Could you check a few things on this model? Use its own coordinates, in mm. Face numbers are marked on the shaded views. Round coordinates to 2 decimals unless told otherwise and drop trailing zeros. Write each loop counter-clockwise with the first axis right and the second up, starting at its lowest first coordinate (ties: lowest second). Pieces come first, ordered by that corner, then holes. Notation, with made-up numbers: M 30.25,-22 L 80.25,-22 A19 ccw 80.25,2 Z; hole C -11,-19 d3. An arc over 180 degrees is marked long. One line per question, with ' | ' between items. Start each with the question number.
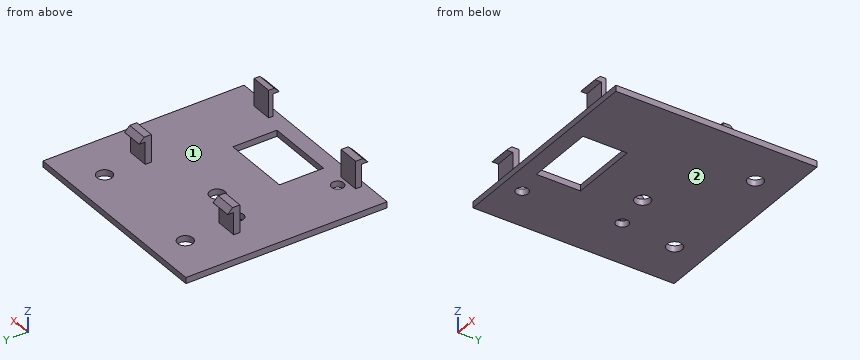
```python
from build123d import *

# Parameters (mm, degrees)
SKETCH_W        = 69
SKETCH_H        = 66
SKETCH_R        = 2.5
SKETCH_R_2      = 2
SKETCH_W_2      = 22.5
SKETCH_H_2      = 14.5
PAD_DEPTH       = 2
SKETCH011_R     = 2.5
POCKET_DEPTH    = 2
SKETCH012_W     = 7
SKETCH012_H     = 2
SKETCH012_H_2   = 1.5
PAD001_DEPTH    = 9
SKETCH013_W     = 7
SKETCH013_H     = 1.7
PAD002_DEPTH    = 2
CHAMFER_SIZE    = 1.65
SKETCH014_W     = 7
SKETCH014_H     = 1.7
PAD003_DEPTH    = 2
CHAMFER001_SIZE = 1.65
SKETCH015_W     = 7
SKETCH015_H     = 1.7
PAD004_DEPTH    = 2
CHAMFER002_SIZE = 1.65
SKETCH016_W     = 7
SKETCH016_H     = 1.7
PAD005_DEPTH    = 2
CHAMFER003_SIZE = 1.65


with BuildPart() as part:
    # Sketch → Pad (new body)
    with BuildSketch(Plane.XY):
        Rectangle(SKETCH_W, SKETCH_H)
        with Locations((-19.5, 23)):
            Circle(SKETCH_R, mode=Mode.SUBTRACT)
        with Locations((19.5, 23)):
            Circle(SKETCH_R, mode=Mode.SUBTRACT)
        with Locations((-20.25, -26.5)):
            Circle(SKETCH_R_2, mode=Mode.SUBTRACT)
        with Locations((-17.85, 4.7)):
            Circle(SKETCH_R_2, mode=Mode.SUBTRACT)
        with Locations((0, -20.75)):
            Rectangle(SKETCH_W_2, SKETCH_H_2, mode=Mode.SUBTRACT)
    extrude(amount=PAD_DEPTH)

    # Sketch011 → Pocket (cut)
    with BuildSketch(Plane.XY.offset(2)):
        with Locations((-5.5, 3)):
            Circle(SKETCH011_R)
    extrude(amount=-POCKET_DEPTH, mode=Mode.SUBTRACT)

    # Sketch012 (on Face5 of Pocket) → Pad001 (join)
    with BuildSketch(Plane.XY.offset(2)):
        with Locations((-21, 9.5)):
            Rectangle(SKETCH012_W, SKETCH012_H)
        with Locations((21, -30.25)):
            Rectangle(SKETCH012_W, SKETCH012_H_2)
        with Locations((21, 10)):
            Rectangle(SKETCH012_W, SKETCH012_H)
        with Locations((-21, -30.5)):
            Rectangle(SKETCH012_W, SKETCH012_H)
    extrude(amount=PAD001_DEPTH)

    # Sketch013 (on Face22 of Pad001) → Pad002 (join)
    with BuildSketch(Plane.XZ.offset(31.5)):
        with Locations((-21, 10.15)):
            Rectangle(SKETCH013_W, SKETCH013_H)
    extrude(amount=PAD002_DEPTH)

    # Chamfer
    chamfer_edges = [part.edges().sort_by_distance(p)[0] for p in [
        (-21, -33.5, 11),
    ]]
    chamfer(chamfer_edges, length=CHAMFER_SIZE)

    # Sketch014 (on Face32 of Chamfer) → Pad003 (join)
    with BuildSketch(Plane.XZ.offset(31)):
        with Locations((21, 10.15)):
            Rectangle(SKETCH014_W, SKETCH014_H)
    extrude(amount=PAD003_DEPTH)

    # Chamfer001
    chamfer001_edges = [part.edges().sort_by_distance(p)[0] for p in [
        (21, -33, 11),
    ]]
    chamfer(chamfer001_edges, length=CHAMFER001_SIZE)

    # Sketch015 (on Face16 of Pad001) → Pad004 (join)
    with BuildSketch(Plane(origin=(0, 11, 0), x_dir=(-1, 0, 0), z_dir=(0, 1, 0))):
        with Locations((-21, 10.15)):
            Rectangle(SKETCH015_W, SKETCH015_H)
    extrude(amount=PAD004_DEPTH)

    # Chamfer002
    chamfer002_edges = [part.edges().sort_by_distance(p)[0] for p in [
        (21, 13, 11),
    ]]
    chamfer(chamfer002_edges, length=CHAMFER002_SIZE)

    # Sketch016 (on Face24 of Chamfer002) → Pad005 (join)
    with BuildSketch(Plane(origin=(0, 10.5, 0), x_dir=(-1, 0, 0), z_dir=(0, 1, 0))):
        with Locations((21, 10.15)):
            Rectangle(SKETCH016_W, SKETCH016_H)
    extrude(amount=PAD005_DEPTH)

    # Chamfer003
    chamfer003_edges = [part.edges().sort_by_distance(p)[0] for p in [
        (-21, 12.5, 11),
    ]]
    chamfer(chamfer003_edges, length=CHAMFER003_SIZE)


solid = part.part
```
1. Suppose I cut it at A-A (z = 3.75). Write out the boundary of the cut face in (x, y).
2. Suppose I cut it at C-C (y = -16.5). Write out the boundary of the cut face in (x, z).
3. If we mould it in two halves opening along Y, with no side actions, what happens to the marked faces 1 and 2? For each: released by +Y, released by -Y, zero draft, split by the parting line, or undercut.
4. Suppose I cut it at D-D (x = 19.5). Write out the boundary of the cut face in (y, z), and give its area (3 significant figures).
5. I'm going to push flat-ended pins straight in: P1, Ø3.5, axis at x = -19.5, z = 5.5, coming from the +Y side; P2, Ø3, axis at y = -32, z = 6, coming from the +X side; P3, Ø4, axis at x = 26.5, z = 2.5, coming from the -Y side. Where does each tip first touch, or does it pass through?
6. I need wall thicknesses on line 1 along Y through (x, z) = (19.5, 1.1); line 2 along Y through (x, z) = (8, 1); line 3 along Y through (x, z) = (-19.5, 1.5). Which ranges of each line are inside material? Lowest first, please. Write a range as from..to.
7. Suppose I cut it at B-B (x = -4). Write out the boundary of the cut face in (y, z).
Computed:
1) outline: M -24.5,-31.5 L -17.5,-31.5 L -17.5,-29.5 L -24.5,-29.5 Z; M -24.5,8.5 L -17.5,8.5 L -17.5,10.5 L -24.5,10.5 Z; M 17.5,-31 L 24.5,-31 L 24.5,-29.5 L 17.5,-29.5 Z; M 17.5,9 L 24.5,9 L 24.5,11 L 17.5,11 Z
2) outline: M -34.5,0 L -11.25,0 L -11.25,2 L -34.5,2 Z; M 11.25,0 L 34.5,0 L 34.5,2 L 11.25,2 Z
3) face 1: undercut | face 2: zero draft
4) outline: M -33,0 L 20.5,0 L 20.5,2 L 11,2 L 11,9.3 L 13,9.3 L 13,9.35 L 11.35,11 L 9,11 L 9,2 L -29.5,2 L -29.5,11 L -31.35,11 L -33,9.35 L -33,9.3 L -31,9.3 L -31,2 L -33,2 Z; M 25.5,0 L 33,0 L 33,2 L 25.5,2 Z | area: 158 mm²
5) P1: stops at y = 10.5 | P2: stops at x = 24.5 | P3: stops at y = -33
6) line 1: y = -33..20.5, 25.5..33 | line 2: y = -33..-28, -13.5..33 | line 3: y = -33..-28.35, -24.65..3.57, 5.83..20.5, 25.5..33
7) outline: M -33,0 L -28,0 L -28,2 L -33,2 Z; M -13.5,0 L 1,0 L 1,2 L -13.5,2 Z; M 5,0 L 33,0 L 33,2 L 5,2 Z
